Verification items for the finished model (mm, model axes). Coordinates: 2 decimals unless noted, no trailing zeros. Write each loop counter-clockwise with the first axis right and the second up, starting at its lowest first coordinate (ties: lowest second). Pieces come first, ordered by that corner, then holes. Notation, with made-up numbers: M -31.5,88 L -22.5,88 A8 ccw -22.5,93 Z; hole C -27.5,-13.75 d9. An arc over 180 degrees is marked long. One line per item, written item: value.
```python
from build123d import *

# Parameters (mm, degrees)
SKETCH1_R           = 2.1
BOSS_EXTRUDE1_DEPTH = 250


with BuildPart() as part:
    # Sketch1 → Boss-Extrude1 (new body)
    with BuildSketch(Plane.XY):
        with BuildLine():
            Line((-2.839339828, 3.9), (-5.470710678, 6.53137085))
            ThreePointArc((-5.470710678, 6.53137085), (-5.492387953, 6.563813185), (-5.5, 6.602081528))
            Line((-5.5, 6.602081528), (-5.5, 8.1))
            ThreePointArc((-5.5, 8.1), (-5.470710678, 8.170710678), (-5.4, 8.2))
            Line((-5.4, 8.2), (-3.334418044, 8.2))
            ThreePointArc((-3.334418044, 8.2), (-3.244178397, 8.256909326), (-3.2566483, 8.362863876))
            Line((-3.2566483, 8.362863876), (-4.58, 10))
            Line((-4.58, 10), (-10, 10))
            Line((-10, 10), (-10, 4.58))
            Line((-10, 4.58), (-8.362863876, 3.2566483))
            ThreePointArc((-8.362863876, 3.2566483), (-8.256909326, 3.244178397), (-8.2, 3.334418044))
            Line((-8.2, 3.334418044), (-8.2, 5.4))
            ThreePointArc((-8.2, 5.4), (-8.170710678, 5.470710678), (-8.1, 5.5))
            Line((-8.1, 5.5), (-6.602081528, 5.5))
            ThreePointArc((-6.602081528, 5.5), (-6.563813185, 5.492387953), (-6.53137085, 5.470710678))
            Line((-6.53137085, 5.470710678), (-3.9, 2.839339828))
            Line((-3.9, 2.839339828), (-3.9, -2.839339828))
            Line((-3.9, -2.839339828), (-6.53137085, -5.470710678))
            ThreePointArc((-6.53137085, -5.470710678), (-6.563813185, -5.492387953), (-6.602081528, -5.5))
            Line((-6.602081528, -5.5), (-8.1, -5.5))
            ThreePointArc((-8.1, -5.5), (-8.170710678, -5.470710678), (-8.2, -5.4))
            Line((-8.2, -5.4), (-8.2, -3.334418044))
            ThreePointArc((-8.2, -3.334418044), (-8.256909326, -3.244178397), (-8.362863876, -3.2566483))
            Line((-8.362863876, -3.2566483), (-10, -4.58))
            Line((-10, -4.58), (-10, -10))
            Line((-10, -10), (-4.58, -10))
            Line((-4.58, -10), (-3.2566483, -8.362863876))
            ThreePointArc((-3.2566483, -8.362863876), (-3.244178397, -8.256909326), (-3.334418044, -8.2))
            Line((-3.334418044, -8.2), (-5.4, -8.2))
            ThreePointArc((-5.4, -8.2), (-5.470710678, -8.170710678), (-5.5, -8.1))
            Line((-5.5, -8.1), (-5.5, -6.602081528))
            ThreePointArc((-5.5, -6.602081528), (-5.492387953, -6.563813185), (-5.470710678, -6.53137085))
            Line((-5.470710678, -6.53137085), (-2.839339828, -3.9))
            Line((-2.839339828, -3.9), (2.839339828, -3.9))
            Line((2.839339828, -3.9), (5.470710678, -6.53137085))
            ThreePointArc((5.470710678, -6.53137085), (5.492387953, -6.563813185), (5.5, -6.602081528))
            Line((5.5, -6.602081528), (5.5, -8.1))
            ThreePointArc((5.5, -8.1), (5.470710678, -8.170710678), (5.4, -8.2))
            Line((5.4, -8.2), (3.334418044, -8.2))
            ThreePointArc((3.334418044, -8.2), (3.244178397, -8.256909326), (3.2566483, -8.362863876))
            Line((3.2566483, -8.362863876), (4.58, -10))
            Line((4.58, -10), (10, -10))
            Line((10, -10), (10, -4.58))
            Line((10, -4.58), (8.362863876, -3.2566483))
            ThreePointArc((8.362863876, -3.2566483), (8.256909326, -3.244178397), (8.2, -3.334418044))
            Line((8.2, -3.334418044), (8.2, -5.4))
            ThreePointArc((8.2, -5.4), (8.170710678, -5.470710678), (8.1, -5.5))
            Line((8.1, -5.5), (6.602081528, -5.5))
            ThreePointArc((6.602081528, -5.5), (6.563813185, -5.492387953), (6.53137085, -5.470710678))
            Line((6.53137085, -5.470710678), (3.9, -2.839339828))
            Line((3.9, -2.839339828), (3.9, 2.839339828))
            Line((3.9, 2.839339828), (6.53137085, 5.470710678))
            ThreePointArc((6.53137085, 5.470710678), (6.563813185, 5.492387953), (6.602081528, 5.5))
            Line((6.602081528, 5.5), (8.1, 5.5))
            ThreePointArc((8.1, 5.5), (8.170710678, 5.470710678), (8.2, 5.4))
            Line((8.2, 5.4), (8.2, 3.334418044))
            ThreePointArc((8.2, 3.334418044), (8.256909326, 3.244178397), (8.362863876, 3.2566483))
            Line((8.362863876, 3.2566483), (10, 4.58))
            Line((10, 4.58), (10, 10))
            Line((10, 10), (4.58, 10))
            Line((4.58, 10), (3.2566483, 8.362863876))
            ThreePointArc((3.2566483, 8.362863876), (3.244178397, 8.256909326), (3.334418044, 8.2))
            Line((3.334418044, 8.2), (5.4, 8.2))
            ThreePointArc((5.4, 8.2), (5.470710678, 8.170710678), (5.5, 8.1))
            Line((5.5, 8.1), (5.5, 6.602081528))
            ThreePointArc((5.5, 6.602081528), (5.492387953, 6.563813185), (5.470710678, 6.53137085))
            Line((5.470710678, 6.53137085), (2.839339828, 3.9))
            Line((2.839339828, 3.9), (-2.839339828, 3.9))
        make_face()
        Circle(SKETCH1_R, mode=Mode.SUBTRACT)
    extrude(amount=BOSS_EXTRUDE1_DEPTH)


solid = part.part
```
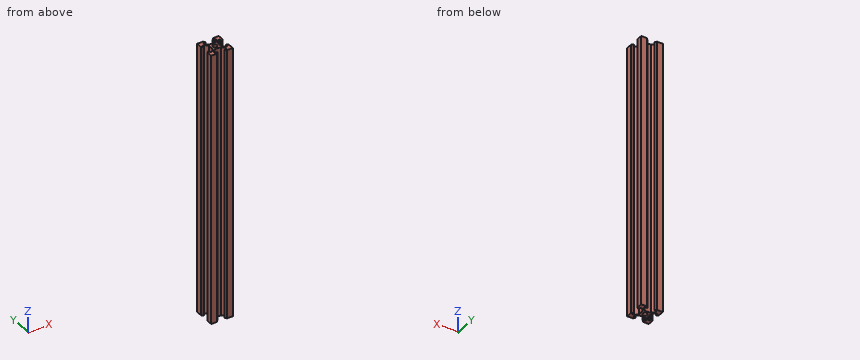
Item 1: Cross-section at A-A, the plane x = 0. Enter the section's corners in (y, z), and give its area (3 significant figures).
The answers:
outline: M -3.9,0 L -2.1,0 L -2.1,250 L -3.9,250 Z; M 2.1,0 L 3.9,0 L 3.9,250 L 2.1,250 Z
area: 900 mm²
Item 2: Go/stop test with flat-tipped pins: P1, Ø6, axis at x = -0.5, z = 106.5, coming from the -Y side; P2, Ø6, axis at y = -1.5, z = 41.5, coming from the +X side; P3, Ø1.7, axis at x = -0.5, z = 86.5, coming from the +Y side. Record where each tip stops, or that it passes through.
The answers:
P1: stops at y = -8.66
P2: stops at x = 9.9
P3: stops at y = 3.9
Item 3: Scan lines: line 1 (Y direction, x = 0, z = 69.5); line 2 (Y direction, x = -8.25, z = 98.5); line 3 (X direction, y = 7.75, z = 142). Record each from-to range of solid material in increasing order.
The answers:
line 1: y = -3.9 to -2.1, 2.1 to 3.9
line 2: y = -10 to -3.25, 3.25 to 10
line 3: x = -10 to -5.5, 5.5 to 10
